from build123d import *

# Parameters (mm, degrees)
BOSS_EXTRUDE1_DEPTH = 3.175
FILLET1_R           = 12.7


with BuildPart() as part:
    # Sketch1 → Boss-Extrude1 (new body)
    with BuildSketch(Plane.XY.offset(1353.875334154)):
        Polygon((-114.199047439, 112.248526419), (-143.93508403, 431.734038744), (143.93508403, 434.29668119), (114.199047439, 114.267866307), align=None)
    extrude(amount=BOSS_EXTRUDE1_DEPTH)

    # Fillet1
    fillet1_edges = [part.edges().sort_by_distance(p)[0] for p in [
        (-114.199047439, 112.248526419, 1355.462834154),
        (-143.93508403, 431.734038744, 1355.462834154),
        (143.93508403, 434.29668119, 1355.462834154),
        (114.199047439, 114.267866307, 1355.462834154),
    ]]
    fillet(fillet1_edges, radius=FILLET1_R)


solid = part.part
Could you check a few things on this model? Use its own coordinates, in mm. Give positions to 0.01 mm unless a question says otherwise; leave off trailing zeros. Loops run counter-clockwise (first coordinate to the right, second up) from the corner with the lowest first, then second, coordinate; pieces in that order, holes last. Notation, with made-up numbers: (62, 72) -> (106, 72) arc R10 ccw to (106, 84) -> close; hole circle Ø11 at (-9.75, 35.25). An arc over 180 degrees is marked (long way). Answer as CSV lines item,"result". Start each with the question number.
(1) If we section it at C-C on y = 240.5: Write out the boundary of the cut face in (x, z), then the cut area to 3 significant figures.
(2) If we section it at A-A on z = 1355.7: Write out the boundary of the cut face in (x, y), then the cut area to 3 significant figures.
(3) I need wall thicknesses on probe 1 along Y at (x, z) = (-111, 1354); probe 2 along Y at (x, z) = (-96, 1354.1); probe 3 along X at (y, z) = (178, 1355.4). Which ranges of each line are inside material? Lowest first, please.
(4) If we section it at B-B on y = 145.5: Write out the boundary of the cut face in (x, z), then the cut area to 3 significant figures.
(5) I'm going to push flat-ended pins straight in: pin 1 Ø1.5 at (y, z) = (213.5, 1354.5) entering from -X; pin 2 Ø1 at (y, z) = (174, 1355) entering from -X. Where does each tip first touch, or does it pass through?
Computed:
1,outline,"(-126.14, 1353.88) -> (125.93, 1353.88) -> (125.93, 1357.05) -> (-126.14, 1357.05) -> close"
1,area,"800 mm2"
2,outline,"(-142.65, 417.98) -> (-115.28, 123.87) arc R12.7 ccw to (-102.52, 112.35) -> (102.73, 114.17) arc R12.7 ccw to (115.26, 125.69) -> (142.63, 420.3) arc R12.7 ccw to (129.88, 434.17) -> (-130.12, 431.86) arc R12.7 ccw to start"
2,area,"82,400 mm2"
3,probe 1,"y = 115.49 to 432.03"
3,probe 2,"y = 112.41 to 432.16"
3,probe 3,"x = -120.32 to 120.12"
4,outline,"(-117.29, 1353.88) -> (117.1, 1353.88) -> (117.1, 1357.05) -> (-117.29, 1357.05) -> close"
4,area,"744 mm2"
5,pin 1,"stops at x = -123.69"
5,pin 2,"stops at x = -119.99"
